```python
from build123d import *

# Parameters (mm, degrees)
SKETCH1_R               = 8.895
BOSS_EXTRUDE1_DEPTH     = 25
CUT_EXTRUDE1_DEPTH      = 12.5
SKETCH3_R               = 1.984375
CUT_EXTRUDE2_DEPTH      = 9.895
CUT_EXTRUDE2_DEPTH_BACK = 9.895


with BuildPart() as part:
    # Sketch1 → Boss-Extrude1 (new body)
    with BuildSketch(Plane(origin=(0, 0, 0), x_dir=(1, 0, 0), z_dir=(0, 1, 0))):
        Circle(SKETCH1_R)
    extrude(amount=-BOSS_EXTRUDE1_DEPTH)

    # Sketch2 → Cut-Extrude1 (cut)
    with BuildSketch(Plane.XZ.offset(25)):
        with BuildLine():
            Line((-6.83125, 1.984375), (-6.83125, -1.984375))
            Line((-6.83125, -1.984375), (-8.670829306, -1.984375))
            ThreePointArc((-8.670829306, -1.984375), (-8.895, 0), (-8.670829306, 1.984375))
            Line((-8.670829306, 1.984375), (-6.83125, 1.984375))
        make_face()
    cut_extrude1 = extrude(amount=-CUT_EXTRUDE1_DEPTH, mode=Mode.SUBTRACT)

    # Mirror1: Cut-Extrude1 across plane
    add(cut_extrude1.mirror(Plane(origin=(0, 0, 0), x_dir=(0, 0, 1), z_dir=(1, 0, 0))), mode=Mode.SUBTRACT)

    # Sketch3 → Cut-Extrude2 (cut, two sides)
    with BuildSketch(Plane(origin=(0, 0, 0), x_dir=(0, 0, -1), z_dir=(1, 0, 0))) as cut_extrude2_sk:
        with Locations((0, -12.5)):
            Circle(SKETCH3_R)
    extrude(amount=CUT_EXTRUDE2_DEPTH, mode=Mode.SUBTRACT)
    extrude(cut_extrude2_sk.sketch, amount=-CUT_EXTRUDE2_DEPTH_BACK, mode=Mode.SUBTRACT)


solid = part.part
```
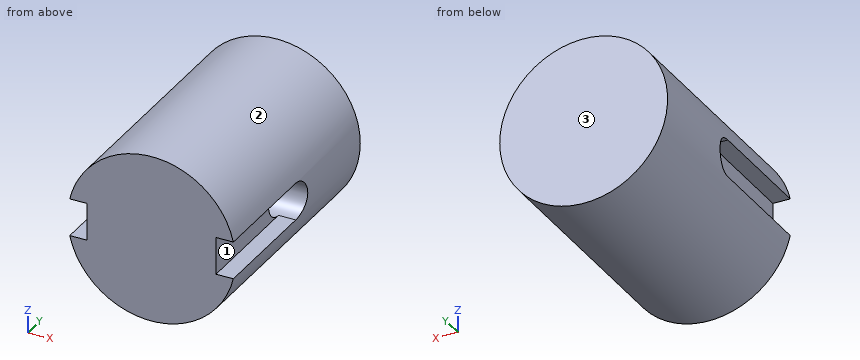
Geometry check sheet. Reference: the model listing, model coordinates, mm. Face numbers are marked on the shaded views. Give positions to 0.01 mm unless a question says otherwise; leave off trailing zeros. Loops run counter-clockwise (first coordinate to the right, second up) from the corner with the lowest first, then second, coordinate; pieces in that order, holes last. Notation, with made-up numbers: M 42.5,79 L 83.5,79 A20 ccw 83.5,84 Z; hole C 43.5,-22.5 d1. An arc over 180 degrees is marked long. Write item = value, one per line. Start each with the question number.
1. Section check A-A, the plane z = 0. Enter the section's corners in (x, y) (3 decimals).
2. Go/stop test with flat-tipped pins: P1, Ø5, axis at y = -12.5, z = 0, coming from the +X side (3 decimals); P2, Ø4.5, axis at y = -21, z = 0.5, coming from the +X side; P3, Ø2, axis at x = -8, y = -17, coming from the -Z side; P4, Ø2, axis at x = 3.5, y = -20, coming from the -Z side. Record where each tip stops, or that it passes through.
3. Thickness scan on probe 1 along Y at (x, z) = (-1.75, 0); probe 2 along Z at (x, y) = (-2, -9.75); probe 3 along Z at (x, y) = (6.25, -12.5). Record the ranges inside material, lowest first.
4. Section check B-B, the plane y = -15.75. Enter the section's corners in (x, z) (3 decimals), plus the area to 3 significant figures.
5. Section check C-C, the plane x = 3.75. Enter the section's corners in (y, z).
6. Draft check along Z on the marked faces 1, 2 and 3. Enter one of: +Z half, -Z half, draft (parallel to the pull), parting line (faces both ways), or undercut.
7. Section check D-D, the plane x = 7.5. Enter the section's corners in (y, z), plus the area to 3 significant figures.
Values follow:
q1.outline = M -8.895,-10.516 L 8.895,-10.516 L 8.895,0 L -8.895,0 Z; M -6.831,-25 L 6.831,-25 L 6.831,-14.484 L -6.831,-14.484 Z
q2.P1 = 8.895
q2.P2 = 8.67
q2.P3 = -5.49
q2.P4 = -8.54
q3.probe_1 = -25 to -14.48, -10.52 to 0
q3.probe_2 = -8.67 to 8.67
q3.probe_3 = -6.33 to -1.98, 1.98 to 6.33
q4.outline = M -8.671,-1.984 A8.895 ccw 8.671,-1.984 L 6.831,-1.984 L 6.831,1.984 L 8.671,1.984 A8.895 ccw -8.671,1.984 L -6.831,1.984 L -6.831,-1.984 Z
q4.area = 233 mm^2
q5.outline = M -25,-8.07 L 0,-8.07 L 0,8.07 L -25,8.07 Z; hole C -12.5,0 d3.97
q6.face_1 = undercut
q6.face_2 = parting line
q6.face_3 = draft
q7.outline = M -25,-4.78 L 0,-4.78 L 0,4.78 L -25,4.78 L -25,1.98 L -12.5,1.98 A1.98 cw -12.5,-1.98 L -25,-1.98 Z
q7.area = 183 mm^2
